from build123d import *

# Parameters (mm, degrees)
CROQUIS1_W              = 22
CROQUIS1_H              = 12
SALIENTE_EXTRUIR1_DEPTH = 22
CROQUIS2_W              = 14
CROQUIS2_H              = 12
SALIENTE_EXTRUIR2_DEPTH = 5
CROQUIS3_R              = 2.5
SALIENTE_EXTRUIR3_DEPTH = 3


with BuildPart() as part:
    # Croquis1 → Saliente-Extruir1 (new body)
    with BuildSketch(Plane(origin=(0, 0, 0), x_dir=(1, 0, 0), z_dir=(0, 1, 0))):
        Rectangle(CROQUIS1_W, CROQUIS1_H)
    extrude(amount=SALIENTE_EXTRUIR1_DEPTH)

    # Croquis2 → Saliente-Extruir2 (add)
    with BuildSketch(Plane(origin=(0, 22, 0), x_dir=(1, 0, 0), z_dir=(0, 1, 0))):
        with Locations((4, 0)):
            Rectangle(CROQUIS2_W, CROQUIS2_H)
    extrude(amount=SALIENTE_EXTRUIR2_DEPTH)

    # Croquis3 → Saliente-Extruir3 (add)
    with BuildSketch(Plane(origin=(0, 27, 0), x_dir=(1, 0, 0), z_dir=(0, 1, 0))):
        with Locations(Location((4, 0, 0), (0, 0, 270))):
            Circle(CROQUIS3_R)
    extrude(amount=SALIENTE_EXTRUIR3_DEPTH)


solid = part.part
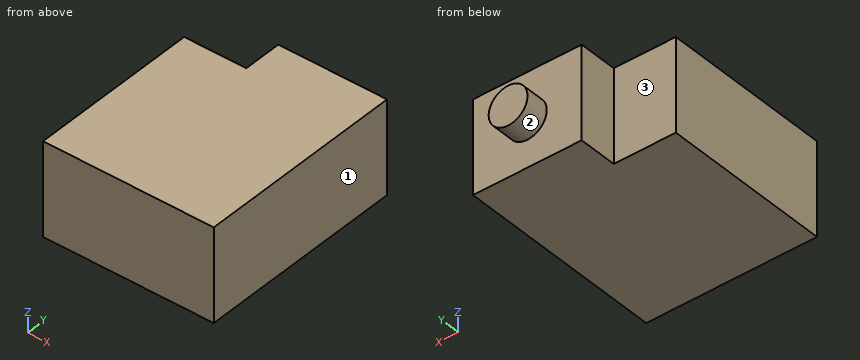
Work out the finished part from the listing and answer in its coordinate system (mm). Face numbers are marked on the shaded views. A direction names the side the tool comes from. Round coordinates to 2 decimals unless told otherwise and drop trailing zeros. Write each loop counter-clockwise with the first axis right and the second up, starting at its lowest first coordinate (ties: lowest second). Pieces come first, ordered by that corner, then holes. Notation, with made-up numbers: (68.25, 9.5) -> (76.25, 9.5) arc R17 cw to (76.25, 17.5) -> close; hole circle Ø10 at (19.25, 49.25). An arc over 180 degrees is marked (long way). Write each question's results on one line, items separated by ' | '.
Item 1: A cutting plane is placed at B-B, the plane z = 0. Determine the outline of the cut face in (x, y), plus the area to 3 significant figures.
Result set:
outline: (-11, 0) -> (11, 0) -> (11, 27) -> (6.5, 27) -> (6.5, 30) -> (1.5, 30) -> (1.5, 27) -> (-3, 27) -> (-3, 22) -> (-11, 22) -> close | area: 569 mm^2
Item 2: A cutting plane is placed at C-C, the plane y = 25.75. Determine the outline of the cut face in (x, z), plus the area to 3 significant figures.
Result set:
outline: (-3, -6) -> (11, -6) -> (11, 6) -> (-3, 6) -> close | area: 168 mm^2
Item 3: A flat-ended cylindrical pin translates along its axis: P1, Ø3, axis at y = 27, z = 1, coming from the -X side. Find the tip coordinate at first contact, or state that the pin passes through.
Result set:
P1: x = -3
Item 4: Which of the six approach directions +Z, -Z, +X, -X, +Y, -Y give full straight-line access (tool end or side, diameter ignored) to the marked faces 1, 2 and 3?
Result set:
face 1: +Z, -Z, +X, +Y, -Y | face 2: +Y | face 3: +Z, -Z, -X, +Y
Item 5: A cutting plane is placed at D-D, the plane x = -8.25. Determine the outline of the cut face in (y, z), plus the area to 3 significant figures.
Result set:
outline: (0, -6) -> (22, -6) -> (22, 6) -> (0, 6) -> close | area: 264 mm^2
Item 6: A cutting plane is placed at A-A, the plane x = 4. Determine the outline of the cut face in (y, z), plus the area to 3 significant figures.
Result set:
outline: (0, -6) -> (27, -6) -> (27, -2.5) -> (30, -2.5) -> (30, 2.5) -> (27, 2.5) -> (27, 6) -> (0, 6) -> close | area: 339 mm^2
Item 7: Find the intervals of material crossed by line 1 along Y through (x, z) = (10, 4); line 2 along X through (y, z) = (24, -0.75); line 3 along Y through (x, z) = (-7.25, -1), in increasing order. Write a range as [from, to].
Result set:
line 1: [0, 27] | line 2: [-3, 11] | line 3: [0, 22]
